```python
from build123d import *

# Parameters (mm, degrees)
PAD_DEPTH    = 3.75
PAD001_DEPTH = 1.25
FILLET_R     = 1


with BuildPart() as part:
    # Sketch → Pad (new body, symmetric)
    with BuildSketch(Plane.XY):
        with BuildLine():
            Line((-5, 0), (-3.75, 0))
            Line((-3.75, 0), (-3.75, 5))
            ThreePointArc((-0.75, 8), (-2.87132, 7.12132), (-3.75, 5))
            Line((-0.75, 8), (0.75, 8))
            ThreePointArc((3.75, 5), (2.87132, 7.12132), (0.75, 8))
            Line((3.75, 5), (3.75, 0))
            Line((3.75, 0), (5, 0))
            Line((5, 0), (5, 5))
            ThreePointArc((5, 5), (3.755204, 8.005204), (0.75, 9.25))
            Line((-0.75, 9.25), (0.75, 9.25))
            ThreePointArc((-0.75, 9.25), (-3.755204, 8.005204), (-5, 5))
            Line((-5, 0), (-5, 5))
        make_face()
    extrude(amount=PAD_DEPTH, both=True)

    # Sketch001 (on Face14 of Pad) → Pad001 (join)
    with BuildSketch(Plane.XY.offset(3.75)):
        with BuildLine():
            Line((-5, 0), (-3.75, 0))
            Line((-3.75, 0), (3.75, 0))
            Line((3.75, 0), (5, 0))
            Line((5, 0), (5, 5))
            ThreePointArc((5, 5), (3.755204, 8.005204), (0.75, 9.25))
            Line((-0.75, 9.25), (0.75, 9.25))
            ThreePointArc((-0.75, 9.25), (-3.755204, 8.005204), (-5, 5))
            Line((-5, 0), (-5, 5))
        make_face()
    pad001 = extrude(amount=PAD001_DEPTH)

    # Mirrored: Pad001 across XY
    add(pad001.mirror(Plane.XY))

    # Fillet
    fillet_edges = [part.edges().sort_by_distance(p)[0] for p in [
        (5, 2.5, 5),
        (5, 2.5, -5),
    ]]
    fillet(fillet_edges, radius=FILLET_R)


solid = part.part
```
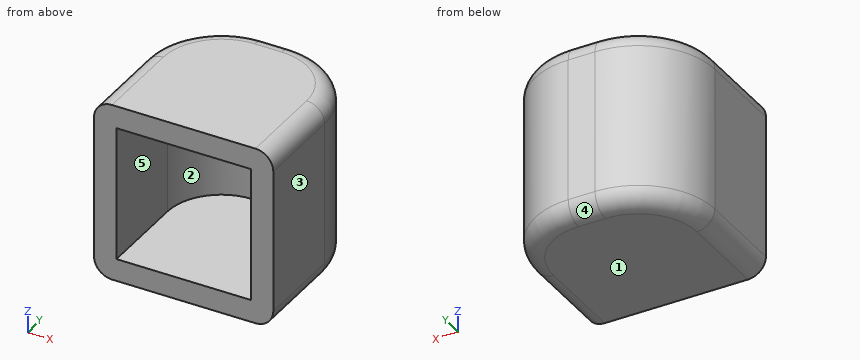
For this review, take the finished solid that the model builds, in its own axes (mm). Face numbers are marked on the shaded views. A direction names the side the tool comes from. Round coordinates to 2 decimals unless told otherwise and drop trailing zeros. Write each loop counter-clockwise with the first axis right and the second up, starting at its lowest first coordinate (ties: lowest second). Pieces come first, ordered by that corner, then holes.
1) Insertion check: pin 1 Ø3 at (x, z) = (2, -2.5) entering from -Y; pin 2 Ø1 at (y, z) = (7, -1.5) entering from +X; pin 3 Ø1.5 at (y, z) = (8, 4) entering from +X; pin 4 Ø3 at (y, z) = (7, 0.5) entering from -X. Each pin has a flat end and moves straight along its axis. Give the tip position at first contact, or say it passes through.
Answer below:
pin 1: stops at y = 0
pin 2: stops at x = 4.73
pin 3: stops at x = 4.36
pin 4: stops at x = -4.97
2) Take a section at C-C on x = 0. Give the boundary of the cut face in (y, z).
Answer below:
outline: (0, -5) - (8.25, -5) arc R1 ccw to (9.25, -4) - (9.25, 4) arc R1 ccw to (8.25, 5) - (0, 5) - (0, 3.75) - (8, 3.75) - (8, -3.75) - (0, -3.75) - close
3) Take a section at B-B on z = 1.5. Give the boundary of the cut face in (x, y), then the cut area to 3 significant figures.
Answer below:
outline: (-5, 0) - (-3.75, 0) - (-3.75, 5) arc R3 cw to (-0.75, 8) - (0.75, 8) arc R3 cw to (3.75, 5) - (3.75, 0) - (5, 0) - (5, 5) arc R4.25 ccw to (0.75, 9.25) - (-0.75, 9.25) arc R4.25 ccw to (-5, 5) - close
area: 28.6 mm2
4) Machinability: for the marked faces 4 and 5, which of the approach directions +Z, -Z, +X, -X, +Y, -Y give a long, thin tool a straight path to every point of the face, cutting with its end or side? Answer none if there is none.
Answer below:
face 4: -Z, +X, -X, +Y
face 5: -Y
5) Mouldability with a two-part tool opening along Z and no side actions: class the marked faces 1, 2 and 3 as +Z half, -Z half, draft (parallel to the pull), parting line (faces both ways), or undercut.
Answer below:
face 1: -Z half
face 2: undercut
face 3: draft
6) Take a section at D-D on z = 4.25. Give the boundary of the cut face in (x, y), then the cut area to 3 significant figures.
Answer below:
outline: (-4.97, 0) - (4.97, 0) - (4.97, 5) arc R4.22 ccw to (0.75, 9.22) - (-0.75, 9.22) arc R4.22 ccw to (-4.97, 5) - close
area: 84.0 mm2
7) For line 1 along X through (y, z) = (5, -1.5), list the stretches that pass through material, from the lowest coordinate up.
Answer below:
line 1: x = -5 to -3.75, 3.75 to 5
8) Take a section at A-A on y = 3.75. Give the boundary of the cut face in (x, z).
Answer below:
outline: (-5, -4) arc R1 ccw to (-4, -5) - (4, -5) arc R1 ccw to (5, -4) - (5, 4) arc R1 ccw to (4, 5) - (-4, 5) arc R1 ccw to (-5, 4) - close; hole (-3.75, -3.75) - (3.75, -3.75) - (3.75, 3.75) - (-3.75, 3.75) - close
